Part model, mm, in its own coordinate system. A direction names the side the tool comes from. Give positions to 0.01 mm unless a question says otherwise; leave off trailing zeros. Loops run counter-clockwise (first coordinate to the right, second up) from the corner with the lowest first, then second, coordinate; pieces in that order, holes last. Notation, with made-up numbers: M 14,24 L 62,24 A26 ccw 62,48 Z; hole C 52.5,48.5 d9. An arc over 180 degrees is marked long. Put each result on its own line as item: value. Start each with the question number.
```python
from build123d import *

# Parameters (mm, degrees)
SKETCH1_W           = 47.09116882
SKETCH1_H           = 77.09116882
BOSS_EXTRUDE1_DEPTH = 1.5
SKETCH2_W           = 44.545584412
SKETCH2_H           = 74.545584412
SKETCH2_W_2         = 42
SKETCH2_H_2         = 72
BOSS_EXTRUDE2_DEPTH = 1.8
FILLET1_R           = 1
SKETCH3_W           = 24
SKETCH3_H           = 64
BOSS_EXTRUDE3_DEPTH = 10
SKETCH4_W           = 48
SKETCH4_H           = 6
CUT_EXTRUDE1_DEPTH  = 24
FILLET2_R           = 6
FILLET3_R           = 1


with BuildPart() as part:
    # Sketch1 → Boss-Extrude1 (new body)
    with BuildSketch(Plane(origin=(0, 0, 0), x_dir=(1, 0, 0), z_dir=(0, 1, 0))):
        with Locations((23.54558441, -38.54558441)):
            Rectangle(SKETCH1_W, SKETCH1_H)
    extrude(amount=BOSS_EXTRUDE1_DEPTH)

    # Sketch2 → Boss-Extrude2 (add)
    with BuildSketch(Plane(origin=(0, 1.5, 0), x_dir=(1, 0, 0), z_dir=(0, 1, 0))):
        with Locations((23.545584412, -38.545584412)):
            Rectangle(SKETCH2_W, SKETCH2_H)
        with Locations((23.545584412, -38.545584412)):
            Rectangle(SKETCH2_W_2, SKETCH2_H_2, mode=Mode.SUBTRACT)
    extrude(amount=BOSS_EXTRUDE2_DEPTH)

    # Fillet1
    fillet1_edges = [part.edges().sort_by_distance(p)[0] for p in [
        (1.272792206, 2.4, 1.272792206),
        (1.272792206, 2.4, 75.818376618),
        (45.818376618, 2.4, 75.818376618),
        (45.818376618, 2.4, 1.272792206),
        (44.545584412, 2.4, 74.545584412),
        (44.545584412, 2.4, 2.545584412),
        (2.545584412, 2.4, 2.545584412),
        (2.545584412, 2.4, 74.545584412),
        (0, 0.75, 0),
        (47.09116882, 0.75, 0),
        (47.09116882, 0.75, 77.09116882),
        (0, 0.75, 77.09116882),
    ]]
    fillet(fillet1_edges, radius=FILLET1_R)

    # Sketch3 → Boss-Extrude3 (add)
    with BuildSketch(Plane.XZ):
        with Locations((23.54558441, 38.542813716)):
            Rectangle(SKETCH3_W, SKETCH3_H)
    extrude(amount=BOSS_EXTRUDE3_DEPTH)

    # Sketch4 → Cut-Extrude1 (cut)
    with BuildSketch(Plane.ZY.offset(-11.54558441)):
        with Locations((38.542813716, -3)):
            Rectangle(SKETCH4_W, SKETCH4_H)
    extrude(amount=-CUT_EXTRUDE1_DEPTH, mode=Mode.SUBTRACT)

    # Fillet2
    fillet2_edges = [part.edges().sort_by_distance(p)[0] for p in [
        (23.54558441, -10, 70.542813716),
        (23.54558441, -10, 6.542813716),
    ]]
    fillet(fillet2_edges, radius=FILLET2_R)

    # Fillet3
    fillet3_edges = [part.edges().sort_by_distance(p)[0] for p in [
        (23.54558441, -6, 14.542813716),
        (23.54558441, -6, 62.542813716),
    ]]
    fillet(fillet3_edges, radius=FILLET3_R)


solid = part.part
```
1) Which spindle directions (+Z, -Z, +X, -X, +Y, -Y) get a long thin tool onto all of the face, cutting with end or side? Do faces 1 (the flat face through (23, -2, 6.543)), 2 (the flat face through (23, -3, 14.543)), 3 (the flat face through (23, 1.5, 38)). Say none if no direction does.
2) Band-saw the part on A-A on z = 51.5. Give the cut face in (x, y).
3) Band-saw the part on C-C on y = -1.75. Give the cut face in (x, z), then the cut area to 3 significant figures.
4) Mould opens along Y. For faces 4 (the flat face through (23, 0, 38)), 5 (the flat face through (1.273, 2, 39)), 6 (the cylindrical face through (23.714, -8.196, 8.254)) say: +Y half, -Y half, draft (parallel to the pull), parting line (faces both ways), or undercut.
5) Wall check: L1, parallel to Y at x = 22.5, z = 61.5; L2, parallel to Z at x = 23.5, y = 2.75; L3, parallel to Z at x = 26, y = -1.75. Give the ranges that are in metal, low to high.
6) Pin check, flat tips, straight feed: pin 1 Ø1.4 at (x, y) = (22, 2.5) entering from -Z; pin 2 Ø2 at (x, y) = (19.5, 3) entering from +Z; pin 3 Ø1 at (y, z) = (-5.5, 64) entering from -X. Stop position of each tip, or through.
7) Band-saw the part on D-D on y = 2.5. Give the cut face in (x, z).
8) Band-saw the part on B-B on x = 14.5. Give the cut face in (y, z).
Evaluation:
1. face 1: -Z, +X, -X, -Y
1. face 2: +X, -X
1. face 3: +Y
2. outline: M 0,0 L 47.09,0 L 47.09,1.5 L 45.82,1.5 L 45.82,3.3 L 44.55,3.3 L 44.55,1.5 L 2.55,1.5 L 2.55,3.3 L 1.27,3.3 L 1.27,1.5 L 0,1.5 Z; M 11.55,-10 L 35.55,-10 L 35.55,-6 L 11.55,-6 Z
3. outline: M 11.55,6.54 L 35.55,6.54 L 35.55,14.54 L 11.55,14.54 Z; M 11.55,62.54 L 35.55,62.54 L 35.55,70.54 L 11.55,70.54 Z
3. area: 384 mm2
4. face 4: undercut
4. face 5: draft
4. face 6: -Y half
5. L1: -10 to -6, 0 to 1.5
5. L2: 1.27 to 2.55, 74.55 to 75.82
5. L3: 6.54 to 14.54, 62.54 to 70.54
6. pin 1: z = 1.27
6. pin 2: z = 75.82
6. pin 3: x = 11.55
7. outline: M 1.27,2.27 A1 ccw 2.27,1.27 L 44.82,1.27 A1 ccw 45.82,2.27 L 45.82,74.82 A1 ccw 44.82,75.82 L 2.27,75.82 A1 ccw 1.27,74.82 Z; hole M 2.55,3.55 A1 ccw 3.55,2.55 L 43.55,2.55 A1 ccw 44.55,3.55 L 44.55,73.55 A1 ccw 43.55,74.55 L 3.55,74.55 A1 ccw 2.55,73.55 Z
8. outline: M -10,12.54 A6 ccw -4,6.54 L 0,6.54 L 0,0 L 1.5,0 L 1.5,1.27 L 3.3,1.27 L 3.3,2.55 L 1.5,2.55 L 1.5,74.55 L 3.3,74.55 L 3.3,75.82 L 1.5,75.82 L 1.5,77.09 L 0,77.09 L 0,70.54 L -4,70.54 A6 ccw -10,64.54 Z; hole M -6,15.54 A1 ccw -5,14.54 L 0,14.54 L 0,62.54 L -5,62.54 A1 ccw -6,61.54 Z
